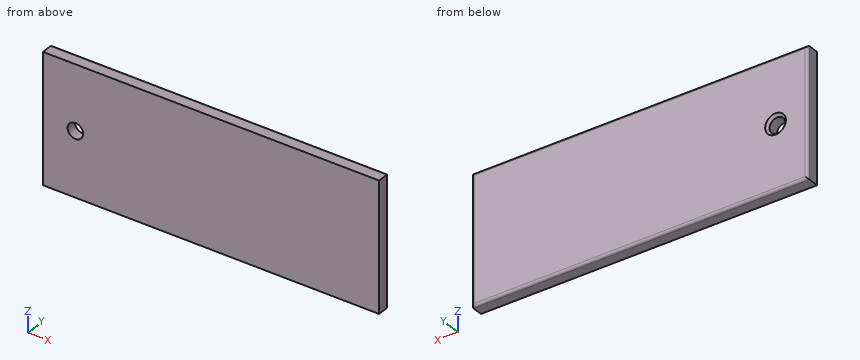
```python
from build123d import *

# Parameters (mm, degrees)
SKETCH1_W           = 260
SKETCH1_H           = 100
BOSS_EXTRUDE1_DEPTH = 10
FILLET1_R           = 2
SKETCH2_R           = 6
CUT_EXTRUDE1_DEPTH  = 140.642400438
CHAMFER1_SIZE       = 2


with BuildPart() as part:
    # Sketch1 → Boss-Extrude1 (new body)
    with BuildSketch(Plane(origin=(0, 0, 0), x_dir=(1, 0, 0), z_dir=(0, 1, 0))):
        Rectangle(SKETCH1_W, SKETCH1_H)
    extrude(amount=BOSS_EXTRUDE1_DEPTH)

    # Fillet1
    fillet1_edges = [part.edges().sort_by_distance(p)[0] for p in [
        (130, 10, 0),
        (0, 10, -50),
        (-130, 10, 0),
        (0, 10, 50),
    ]]
    fillet(fillet1_edges, radius=FILLET1_R)

    # Sketch2 → Cut-Extrude1 (cut, through all)
    with BuildSketch(Plane(origin=(0, 10, 0), x_dir=(1, 0, 0), z_dir=(0, 1, 0))):
        with Locations(Location((-105, 0, 0), (0, 0, 270))):
            Circle(SKETCH2_R)
    extrude(amount=-CUT_EXTRUDE1_DEPTH, mode=Mode.SUBTRACT)

    # Chamfer1
    chamfer1_edges = [part.edges().sort_by_distance(p)[0] for p in [
        (-105, 10, -6),
    ]]
    chamfer(chamfer1_edges, length=CHAMFER1_SIZE)


solid = part.part
```
For this review, take the finished solid that the model builds, in its own axes (mm). Give positions to 0.01 mm unless a question says otherwise; leave off trailing zeros. Write each loop counter-clockwise with the first axis right and the second up, starting at its lowest first coordinate (ties: lowest second). Pieces come first, ordered by that corner, then holes. Notation, with made-up numbers: M 9,75 L 42,75 A19 ccw 42,94 Z; hole C 85.25,-36 d8. An arc over 180 degrees is marked long. Answer as CSV lines item,"result".
1. Wall thickness on line 1 (X direction, y = 3.75, z = 0); line 2 (X direction, y = 2.25, z = 2); line 3 (X direction, y = 8.75, z = 38.5): over which ranges is each line inside the solid? List them lowest first.
Findings:
line 1,"x = -130 to -111, -99 to 130"
line 2,"x = -130 to -110.66, -99.34 to 130"
line 3,"x = -129.85 to 129.85"
2. Consider section A-A, the plane x = -105. Write out the cut boundary in (y, z), then the cut area to 3 significant figures.
Findings:
outline,"M 0,-50 L 8,-50 A2 ccw 10,-48 L 10,-8 L 8,-6 L 0,-6 Z; M 0,6 L 8,6 L 10,8 L 10,48 A2 ccw 8,50 L 0,50 Z"
area,"874 mm2"
3. Consider section B-B, the plane z = 0. Write out the cut boundary in (x, y), then the cut area to 3 significant figures.
Findings:
outline,"M -130,0 L -111,0 L -111,8 L -113,10 L -128,10 A2 ccw -130,8 Z; M -99,0 L 130,0 L 130,8 A2 ccw 128,10 L -97,10 L -99,8 Z"
area,"2,470 mm2"
